Build history of the part. All positions in model axes, mm. Face numbers are marked on the shaded views. Round coordinates to 2 decimals unless told otherwise and drop trailing zeros. Write each loop counter-clockwise with the first axis right and the second up, starting at its lowest first coordinate (ties: lowest second). Pieces come first, ordered by that corner, then holes. Notation, with made-up numbers: M -37,-23.5 L -7,-23.5 A15 cw -7,-4.5 Z; hole C 62.5,-36.5 d2. An arc over 180 degrees is marked long. Use a Markdown table: item, result.
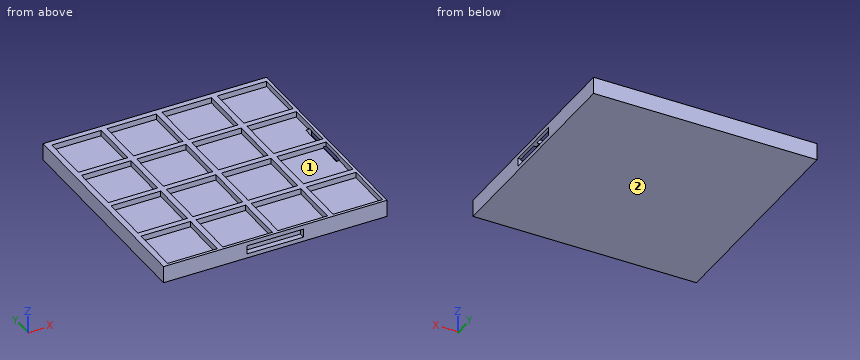
from build123d import *

# Parameters (mm, degrees)
F0_W     = 100.33
F0_H     = 100.33
F1_DEPTH = 7.62
F2_W     = 22.225
F2_H     = 22.225
F3_DEPTH = 2.54
F4_W     = 25.4
F4_H     = 3.81
F6_DEPTH = 2.54
F5_W     = 25.4
F5_H     = 3.81
F7_DEPTH = 2.54


with BuildPart() as f1:
    # F0 (on Top) → F1 (new body)
    with BuildSketch(Plane.XY):
        with Locations((50.165, 50.165)):
            Rectangle(F0_W, F0_H)
    extrude(amount=-F1_DEPTH)

    # F2 (on Top) → F3 (cut)
    with BuildSketch(Plane.XY):
        with Locations((13.6525, 86.6775)):
            Rectangle(F2_W, F2_H)
        with Locations((38.4175, 86.6775)):
            Rectangle(F2_W, F2_H)
        with Locations((63.1825, 86.6775)):
            Rectangle(F2_W, F2_H)
        with Locations((87.9475, 86.6775)):
            Rectangle(F2_W, F2_H)
        with Locations((13.6525, 61.9125)):
            Rectangle(F2_W, F2_H)
        with Locations((13.6525, 37.1475)):
            Rectangle(F2_W, F2_H)
        with Locations((13.6525, 12.3825)):
            Rectangle(F2_W, F2_H)
        with Locations((38.4175, 61.9125)):
            Rectangle(F2_W, F2_H)
        with Locations((63.1825, 61.9125)):
            Rectangle(F2_W, F2_H)
        with Locations((87.9475, 61.9125)):
            Rectangle(F2_W, F2_H)
        with Locations((38.4175, 37.1475)):
            Rectangle(F2_W, F2_H)
        with Locations((38.4175, 12.3825)):
            Rectangle(F2_W, F2_H)
        with Locations((63.1825, 37.1475)):
            Rectangle(F2_W, F2_H)
        with Locations((87.9475, 37.1475)):
            Rectangle(F2_W, F2_H)
        with Locations((63.1825, 12.3825)):
            Rectangle(F2_W, F2_H)
        with Locations((87.9475, 12.3825)):
            Rectangle(F2_W, F2_H)
    extrude(amount=-F3_DEPTH, mode=Mode.SUBTRACT)

    # F4 (on face) → F6 (cut)
    with BuildSketch(Plane.XZ):
        with Locations((50.165, -3.81)):
            Rectangle(F4_W, F4_H)
    extrude(amount=-F6_DEPTH, mode=Mode.SUBTRACT)

    # F5 (on face) → F7 (cut)
    with BuildSketch(Plane.YZ.offset(100.33)):
        with Locations((50.165, -3.81)):
            Rectangle(F5_W, F5_H)
    extrude(amount=-F7_DEPTH, mode=Mode.SUBTRACT)


solid = f1.part
Q1. Cut at C-C on y = 28. Give the cut face in (x, z) (3 decimals), and give its area (3 significant figures).
Response values:
| item | result |
|---|---|
| outline | M 0,-7.62 L 100.33,-7.62 L 100.33,0 L 99.06,0 L 99.06,-2.54 L 76.835,-2.54 L 76.835,0 L 74.295,0 L 74.295,-2.54 L 52.07,-2.54 L 52.07,0 L 49.53,0 L 49.53,-2.54 L 27.305,-2.54 L 27.305,0 L 24.765,0 L 24.765,-2.54 L 2.54,-2.54 L 2.54,0 L 0,0 Z |
| area | 539 mm2 |
Q2. Cut at B-B on x = 84. Give the cut face in (y, z) (3 decimals).
Response values:
| item | result |
|---|---|
| outline | M 0,-7.62 L 100.33,-7.62 L 100.33,0 L 97.79,0 L 97.79,-2.54 L 75.565,-2.54 L 75.565,0 L 73.025,0 L 73.025,-2.54 L 50.8,-2.54 L 50.8,0 L 48.26,0 L 48.26,-2.54 L 26.035,-2.54 L 26.035,0 L 23.495,0 L 23.495,-2.54 L 1.27,-2.54 L 1.27,0 L 0,0 Z |
Q3. Cut at A-A on y = 39.5. Give the cut face in (x, z) (3 decimals), and give its area (3 significant figures).
Response values:
| item | result |
|---|---|
| outline | M 0,-7.62 L 100.33,-7.62 L 100.33,-5.715 L 97.79,-5.715 L 97.79,-2.54 L 76.835,-2.54 L 76.835,0 L 74.295,0 L 74.295,-2.54 L 52.07,-2.54 L 52.07,0 L 49.53,0 L 49.53,-2.54 L 27.305,-2.54 L 27.305,0 L 24.765,0 L 24.765,-2.54 L 2.54,-2.54 L 2.54,0 L 0,0 Z; M 99.06,-1.905 L 100.33,-1.905 L 100.33,0 L 99.06,0 Z |
| area | 530 mm2 |
Q4. Drop flat-ended pins along their axis: P1, Ø0.8, axis at y = 38, z = -0.5, coming from the -X side; P2, Ø1, axis at x = 40.5, y = 59.5, coming from the +Z side. Give the stop position or say it passes through.
Response values:
| item | result |
|---|---|
| P1 | stops at x = 0 |
| P2 | stops at z = -2.54 |
Q5. Two-plate mould, pull along Y, no slides. Class the marked faces 1 and 2: +Y half, -Y half, draft (parallel to the pull), parting line (faces both ways), or undercut.
Response values:
| item | result |
|---|---|
| face 1 | undercut |
| face 2 | draft |
Q6. Drill centre lines: L1, parallel to X at y = 28.5, z = -2.25 (3 decimals); L2, parallel to Y at x = 14, z = -0.25 (3 decimals); L3, parallel to Z at x = 82, y = 90. Where is each one in solid material? Low to high.
Response values:
| item | result |
|---|---|
| L1 | x = 0 to 2.54, 24.765 to 27.305, 49.53 to 52.07, 74.295 to 76.835, 99.06 to 100.33 |
| L2 | y = 0 to 1.27, 23.495 to 26.035, 48.26 to 50.8, 73.025 to 75.565, 97.79 to 100.33 |
| L3 | z = -7.62 to -2.54 |
